from build123d import *

# Parameters (mm, degrees)
SKETCH_2_R             = 4
SKETCH_2_R_2           = 1.7
EXTRUDE_1_DEPTH        = 6
PATTERN_LINEAR_1_COUNT = 2
PATTERN_LINEAR_1_PITCH = 12.5
SKETCH_3_R             = 1.7
EXTRUDE_2_DEPTH        = 18.5
SKETCH_4_R             = 5.5
CUT_EXTRUDE_1_DEPTH    = 6.5
SKETCH_9_W             = 14.956687691
SKETCH_9_H             = 17.867271405
CUT_EXTRUDE_3_DEPTH    = 3.45
CHAMFER_1_SIZE         = 3


with BuildPart() as part:
    # Sketch 2 → Extrude 1 (new body)
    with BuildSketch(Plane.XY):
        Circle(SKETCH_2_R)
        Circle(SKETCH_2_R_2, mode=Mode.SUBTRACT)
    extrude(amount=EXTRUDE_1_DEPTH)


with BuildPart() as pattern_linear_1_1:
    # Pattern Linear 1: pattern copy
    add(part.part.moved(Location(Vector(0, 0, 1) * (1 * PATTERN_LINEAR_1_PITCH))))


with BuildPart() as part_1:
    add(part.part)

    add(pattern_linear_1_1.part)  # Extrude 2 merges Pattern Linear 1_1
    # Sketch 3 → Extrude 2 (add)
    with BuildSketch(Plane(origin=(0, 0, 0), x_dir=(-1, 0, 0), z_dir=(0, 0, -1))):
        with BuildLine():
            Line((3.799671038, 1.25), (25.799671038, 1.25))
            Line((25.799671038, 1.25), (25.799671038, 6.75))
            ThreePointArc((25.799671038, 6.75), (27.049671038, 14.549671038), (28.299671038, 6.75))
            Line((28.299671038, 6.75), (28.299671038, -1.25))
            Line((28.299671038, -1.25), (25.799671038, -1.25))
            Line((25.799671038, -1.25), (3.799671038, -1.25))
            Line((3.799671038, -1.25), (3.799671038, 1.25))
        make_face()
        with Locations((27.049671038, 10.549671038)):
            Circle(SKETCH_3_R, mode=Mode.SUBTRACT)
    extrude(amount=-EXTRUDE_2_DEPTH)

    # Sketch 4 → Cut-Extrude 1 (cut)
    with BuildSketch(Plane.XY.offset(6)):
        Circle(SKETCH_4_R)
    extrude(amount=CUT_EXTRUDE_1_DEPTH, mode=Mode.SUBTRACT)

    # Sketch 9 → Cut-Extrude 3 (cut)
    with BuildSketch(Plane(origin=(0, 0, 9.25), x_dir=(-1, 0, 0), z_dir=(0, 0, -1))):
        with Locations((27.795829792, 10.183635703)):
            Rectangle(SKETCH_9_W, SKETCH_9_H)
    cut_extrude_3 = extrude(amount=CUT_EXTRUDE_3_DEPTH, mode=Mode.SUBTRACT)

    # Mirror 1: Cut-Extrude 3 across plane
    add(cut_extrude_3.mirror(Plane(origin=(0, 0, 9.25), x_dir=(1, 0, 0), z_dir=(0, 0, -1))), mode=Mode.SUBTRACT)

    # Chamfer 1
    chamfer_1_edges = [part_1.edges().sort_by_distance(p)[0] for p in [
        (-25.799671038, 1.25, 15.6),
        (-25.799671038, 1.25, 2.9),
    ]]
    chamfer(chamfer_1_edges, length=CHAMFER_1_SIZE)


solid = part_1.part
Geometry: final body of the model. Coordinates: model frame, mm. A direction names the side the tool comes from. Coordinates: 2 decimals unless noted, no trailing zeros. Order: outer loops, then holes, each group sorted by start corner. A loop starts at its lowest first (then second) coordinate and runs counter-clockwise, first axis right, second up.
1) Section D-D (x = 0). Return loops of the section in (y, z), then the cut area to 3 significant figures.
Result sheet:
outline: (-4, 0) - (-1.7, 0) - (-1.7, 6) - (-4, 6) - close; (-4, 12.5) - (-1.7, 12.5) - (-1.7, 18.5) - (-4, 18.5) - close; (1.7, 0) - (4, 0) - (4, 6) - (1.7, 6) - close; (1.7, 12.5) - (4, 12.5) - (4, 18.5) - (1.7, 18.5) - close
area: 55.2 mm2
2) Set-up query: faces 4 (the cylindrical face through (-5.5, 0, 9.2)), 5 (the flat face through (-24.32, 2.77, 2.86)), 6 (the flat face through (-16, -1.25, 9)), 7 (the flat face through (-27, 8, 5.8)). Return all of +Z, -Z, +X, -X, +Y, -Y with unobstructed straight access to the full face (end or side cutting, diameter ignored); none if empty.
Result sheet:
face 4: +X
face 5: +Z, -Z
face 6: +Z, -Z, -X, -Y
face 7: -X, +Y
3) First-contact query: P1, Ø9, axis at y = 1.5, z = 10, coming from the -X side; P2, Ø2.5, axis at x = -27.05, y = 10.55, coming from the +Z side; P3, Ø2, axis at y = 6, z = 2.5, coming from the +X side; P4, Ø5, axis at x = -9, z = 16.5, coming from the -Y side. Flat tips, straight axial feed; report the tip coordinate or a pass-through.
Result sheet:
P1: stops at x = -28.3
P2: passes through
P3: stops at x = -25.21
P4: stops at y = -1.25
4) Draft query along X for faces 1 (the flat face through (-2, 0, 12.5)), 2 (the flat face through (-16, 1.25, 9)), 3 (the flat face through (-25.8, 5, 16)). Return one class per face: released by +X, released by -X, zero draft, split by the parting line, or undercut.
Result sheet:
face 1: zero draft
face 2: undercut
face 3: released by +X
5) Ray query, probe 1 along Z at (x, y) = (-1, -2.25); probe 2 along Z at (x, y) = (-27.5, 1.75); probe 3 along Y at (x, z) = (0, 2.6). Return the intervals inside material, ascending.
Result sheet:
probe 1: z = 0 to 6, 12.5 to 18.5
probe 2: z = 0 to 5.8, 12.7 to 18.5
probe 3: y = -4 to -1.7, 1.7 to 4
6) Section B-B (x = -4.5). Return loops of the section in (y, z).
Result sheet:
outline: (-1.25, 0) - (1.25, 0) - (1.25, 6) - (-1.25, 6) - close; (-1.25, 12.5) - (1.25, 12.5) - (1.25, 18.5) - (-1.25, 18.5) - close
7) Section A-A (y = 5.5). Return loops of the section in (x, z).
Result sheet:
outline: (-28.3, 0) - (-25.8, 0) - (-25.8, 5.8) - (-28.3, 5.8) - close; (-28.3, 12.7) - (-25.8, 12.7) - (-25.8, 18.5) - (-28.3, 18.5) - close
8) Section C-C (y = 0). Return loops of the section in (x, z).
Result sheet:
outline: (-28.3, 0) - (-1.7, 0) - (-1.7, 6) - (-5.5, 6) - (-5.5, 12.5) - (-1.7, 12.5) - (-1.7, 18.5) - (-28.3, 18.5) - close; (1.7, 0) - (4, 0) - (4, 6) - (1.7, 6) - close; (1.7, 12.5) - (4, 12.5) - (4, 18.5) - (1.7, 18.5) - close
